Input: part model. Units: mm. Frame: model coordinates. Give positions to 0.01 mm unless a question says otherwise; leave off trailing zeros. Loops run counter-clockwise (first coordinate to the right, second up) from the corner with the lowest first, then second, coordinate; pieces in that order, holes last. Notation, with made-up numbers: (89, -16) -> (124, -16) arc R32 cw to (124, 16) -> close; hole circle Ø11 at (-29.5, 49). An arc over 180 degrees is marked (long way). Answer as a JSON object with one key per item and string values.
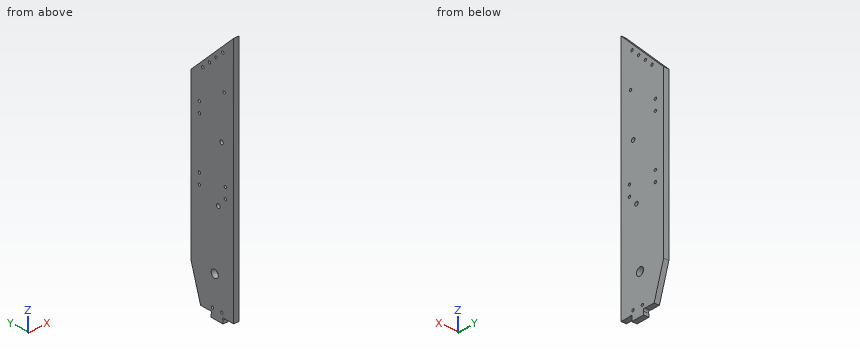
Autodesk Inventor part; units mm, degrees
ref_plane "YZ Plane" through (0, 0, 0) normal (1, 0, 0) x (0, 1, 0)
ref_plane "XZ Plane" through (0, 0, 0) normal (0, 1, 0) x (-1, 0, 0)
ref_plane "XY Plane" through (0, 0, 0) normal (0, 0, 1) x (1, 0, 0)
sketch "Sketch1" plane through (0, 0, 0) normal (1, 0, 0) x (0, 1, 0)
  line L0 (0, 0) -> (101.6, 0)
  line L1 (101.6, 0) -> (101.6, -508)
  line L2 (101.6, -508) -> (0, -508)
  line L3 (0, -508) -> (0, 0)
  line L4 (0, 0) -> (0, 101.6)
  line L5 (0, 101.6) -> (101.6, 0)
  line L6 (101.6, -508) -> (114.3, -508)
  line L7 (114.3, -508) -> (114.3, -12.7)
  line L8 (114.3, -12.7) -> (101.6, -12.7)
  line L9 (101.6, -12.7) -> (101.6, -508)
  line L10 (114.3, -12.7) -> (101.6, 0)
  line L11 (0, -508) -> (28.575, -508)
  line L12 (28.575, -508) -> (28.575, -495.3)
  line L13 (28.575, -495.3) -> (0, -495.3)
  line L14 (0, -495.3) -> (0, -508)
  line L15 (60.325, -508) -> (114.3, -508)
  line L16 (114.3, -508) -> (114.3, -495.3)
  line L17 (114.3, -495.3) -> (60.325, -495.3)
  line L18 (60.325, -495.3) -> (60.325, -508)
  circle A0 centre (50.8, -412.75) radius 9.525
  line L19 (50.8, -412.75) -> (127.2366, -412.75)
  line L20 (114.3, -412.75) -> (88.9, -495.3)
  point P0 (0, -495.3)
  dimension "d0" = 508
  dimension "d1" = 101.6
  dimension "d2" = 101.6
  dimension "d3" = 12.7
  dimension "d4" = 495.3
  dimension "d5" = 28.575
  dimension "d6" = 12.7
  dimension "d7" = 31.75
  dimension "d8" = 19.05
  dimension "d9" = 95.25
  dimension "d10" = 50.8
  dimension "d11" = 28.575
  dimension "d14" = 12.7
extrude "Extrusion1" add sketch "Sketch1" along normal blind 12.7 contours L4 L5 L0 | L0 L1 L20 L17 L18 L2 L12 L13 L3 | L10 L8 L1 | L8 L7 L19 L1 | L19 L20 L1
sketch "Sketch2" plane through (12.7, 0, 0) normal (1, 0, 0) x (0, 0, -1)
  line L0 (508, 60.325) -> (495.3, 60.325)
  line L1 (495.3, 60.325) -> (497.5451, 62.5701)
  line L2 (495.3, 0) -> (495.3, 28.575)
  line L3 (495.3, 28.575) -> (497.5451, 26.3299)
  line L4 (495.3, 28.575) -> (508, 28.575)
  circle A0 centre (497.5451, 62.5701) radius 3.175
  circle A1 centre (497.5451, 26.3299) radius 3.175
  point P0 (0, 0)
  dimension "d15" = 3.175
  dimension "d16" = 45
  dimension "d17" = 3.175
  dimension "d18" = 45
  dimension "d19" = 6.35
  dimension "d20" = 6.35
extrude "Extrusion2" cut sketch "Sketch2" against normal blind 12.7
sketch "Sketch3" plane through (12.7, 0, 0) normal (1, 0, 0) x (0, 0, -1)
  circle A0 centre (485.775, 57.15) radius 3.175
  line L0 (495.3, 64.8151) -> (495.3, 88.9)
  line L1 (508, 28.575) -> (508, 60.325)
  circle A1 centre (485.775, 31.75) radius 3.175
  line L2 (495.3, 0) -> (495.3, 24.0849)
  line L3 (12.7, 114.3) -> (-101.6, 0)
  line L4 (-83.6395, 17.9605) -> (-29.758, 71.842)
  line L5 (-29.758, 71.842) -> (-16.2876, 58.3717)
  line L6 (-16.2876, 58.3717) -> (-70.1691, 4.4901)
  line L7 (-70.1691, 4.4901) -> (-83.6395, 17.9605)
  circle A2 centre (-58.9438, 29.1858) radius 3.175
  circle A3 centre (-40.9833, 47.1463) radius 3.175
  point P0 (0, 0)
  point P1 (508, 44.45)
  point P2 (508, 44.45)
  dimension "d23" = 6.35
  dimension "d25" = 9.525
  dimension "d27" = 12.7
  dimension "d28" = 6.35
  dimension "d29" = 9.525
  dimension "d30" = 12.7
  dimension "d31" = 19.05
  dimension "d32" = 76.2
  dimension "d33" = 25.4
  dimension "d34" = 6.35
  dimension "d35" = 6.35
  dimension "d36" = 9.525
  dimension "d37" = 9.525
  dimension "d38" = 25.4
  dimension "d39" = 25.4
extrude "Extrusion3" cut sketch "Sketch3" against normal blind 12.7 contours A0 | A1 | A2 | A3
sketch "Sketch4" plane through (12.7, 0, 0) normal (1, 0, 0) x (0, 0, -1)
  circle A0 centre (218.821, 92.075) radius 3.175
  line L0 (-101.6, 0) -> (495.3, 0)
  circle A1 centre (244.221, 92.075) radius 3.175
  point P0 (0, 0)
  dimension "d42" = 6.35
  dimension "d43" = 92.075
  dimension "d44" = 6.35
  dimension "d45" = 92.075
  dimension "d46" = 218.821
  dimension "d47" = 244.221
extrude "Extrusion4" cut sketch "Sketch4" against normal blind 12.7
sketch "Sketch6" plane through (12.7, 0, 0) normal (1, 0, 0) x (0, 0, -1)
  circle A0 centre (218.821, 22.225) radius 3.175
  circle A1 centre (244.221, 22.225) radius 3.175
  line L0 (-101.6, 0) -> (495.3, 0)
  point P0 (0, 0)
  dimension "d59" = 6.35
  dimension "d60" = 6.35
  dimension "d61" = 218.821
  dimension "d62" = 22.225
  dimension "d63" = 22.225
  dimension "d64" = 25.4
extrude "Extrusion6" cut sketch "Sketch6" against normal blind 12.7
sketch "Sketch7" plane through (12.7, 0, 0) normal (1, 0, 0) x (0, 0, -1)
  circle A0 centre (69.85, 92.075) radius 3.175
  circle A1 centre (95.25, 92.075) radius 3.175
  line L0 (412.75, 114.3) -> (12.7, 114.3)
  point P0 (0, 0)
  dimension "d67" = 6.35
  dimension "d68" = 6.35
  dimension "d69" = 69.85
  dimension "d70" = 22.225
  dimension "d71" = 22.225
  dimension "d72" = 25.4
extrude "Extrusion7" cut sketch "Sketch7" against normal blind 12.7
sketch "Sketch10" plane through (12.7, 0, 0) normal (1, 0, 0) x (0, 0, -1)
  circle A0 centre (22.225, 25.4) radius 3.175
  line L0 (-101.6, 0) -> (495.3, 0)
  circle A1 centre (412.75, 50.8) radius 9.525
  circle A2 centre (412.75, 50.8) radius 76.2
  circle A3 centre (22.225, 25.4) radius 38.1
  line L1 (22.225, 25.4) -> (412.75, 50.8)
  circle A4 centre (129.9474, 32.4063) radius 4.7625
  circle A5 centre (267.0079, 41.3208) radius 4.7625
  point P0 (0, 0)
  dimension "d82" = 6.35
  dimension "d83" = 25.4
  dimension "d84" = 22.225
  dimension "d85" = 152.4
  dimension "d86" = 76.2
  dimension "d87" = 9.525
  dimension "d88" = 107.95
  dimension "d89" = 9.525
  dimension "d90" = 146.05
extrude "Extrusion8" cut sketch "Sketch10" against normal blind 12.7 contours A0 | A4 L1 | L1 A4 | A5 L1 | L1 A5
sketch "Sketch15" plane through (12.7, 0, 0) normal (1, 0, 0) x (0, 0, -1)
  circle A0 centre (-23.0228, 65.1069) radius 3.175
  line L0 (12.7, 114.3) -> (-101.6, 0)
  circle A1 centre (-40.9833, 47.1463) radius 3.175
  circle A2 centre (-5.0622, 83.0674) radius 3.175
  line L1 (-74.6592, 26.9408) -> (-2.8172, 98.7828)
  line L2 (-2.8172, 98.7828) -> (10.6532, 85.3124)
  line L3 (10.6532, 85.3124) -> (-61.1888, 13.4704)
  line L4 (-61.1888, 13.4704) -> (-74.6592, 26.9408)
  circle A3 centre (-58.9438, 29.1858) radius 3.175
  point P0 (0, 0)
  dimension "d103" = 6.35
  dimension "d104" = 9.525
  dimension "d105" = 25.4
  dimension "d106" = 6.35
  dimension "d107" = 9.525
  dimension "d108" = 25.4
  dimension "d109" = 19.05
  dimension "d110" = 12.7
  dimension "d111" = 101.6
extrude "Extrusion11" cut sketch "Sketch15" against normal blind 12.7 contours A0 | A2
properties part number "Side Wall_outer"
Q1. Section A-A, the plane x = 5. Give the number of separate pieces and of enclosed holes in the cut face, then the cut area to 3 significant figures.
Evaluation:
{"separate pieces": "1", "enclosed holes": "16", "area": "60,200 mm2"}
Q2. Ray query, line 1 along Y through (x, z) = (3, -413); line 2 along Y through (x, z) = (6.75, -95.25); line 3 along Z through (x, y) = (11, 39). Return the intervals inside material, ascending.
Evaluation:
{"line 1": "y = 0 to 41.28, 60.32 to 114.22", "line 2": "y = 0 to 88.9, 95.25 to 114.3", "line 3": "z = -508 to -271.17, -262.85 to 62.6"}
Q3. Section B-B, the plane y = 7.5. Return the cut outline in (x, z).
Evaluation:
{"outline": "(0, -495.3) -> (12.7, -495.3) -> (12.7, 94.1) -> (0, 94.1) -> close"}
Q4. Pin query (flat end, axial travel): pin 1 (3 mm diameter, centred on x = 9.5, y = 87.5, fed in from -Z); pin 2 (6.5 mm diameter, centred on x = 6.5, z = -502.5, fed in from -Y) (3 decimals). Return the tip coordinate at first contact, or that it passes through.
Evaluation:
{"pin 1": "stops at z = -495.3", "pin 2": "stops at y = 28.575"}
